from build123d import *

# Parameters (mm, degrees)
SKETCH1_W           = 9.75
SKETCH1_H           = 9.75
SKETCH1_W_2         = 7.75
SKETCH1_H_2         = 7.75
BOSS_EXTRUDE1_DEPTH = 10
BOSS_EXTRUDE2_DEPTH = 4
FILLET1_R           = 1


with BuildPart() as part:
    # Sketch1 → Boss-Extrude1 (new body)
    with BuildSketch(Plane.XY):
        Rectangle(SKETCH1_W, SKETCH1_H)
        Rectangle(SKETCH1_W_2, SKETCH1_H_2, mode=Mode.SUBTRACT)
    extrude(amount=BOSS_EXTRUDE1_DEPTH)

    # Sketch2 → Boss-Extrude2 (add)
    with BuildSketch(Plane.XY.offset(10)):
        with BuildLine():
            Line((-5.253161089, 7.228716278), (5.253161089, 7.228716278))
            ThreePointArc((5.253161089, 7.228716278), (6.667374652, 6.64292984), (7.253161089, 5.228716278))
            Line((7.253161089, 5.228716278), (7.253161089, -5.228716278))
            ThreePointArc((7.253161089, -5.228716278), (6.667374652, -6.64292984), (5.253161089, -7.228716278))
            Line((5.253161089, -7.228716278), (-5.253161089, -7.228716278))
            ThreePointArc((-5.253161089, -7.228716278), (-6.667374652, -6.64292984), (-7.253161089, -5.228716278))
            Line((-7.253161089, -5.228716278), (-7.253161089, 5.228716278))
            ThreePointArc((-7.253161089, 5.228716278), (-6.667374652, 6.64292984), (-5.253161089, 7.228716278))
        make_face()
    extrude(amount=BOSS_EXTRUDE2_DEPTH)

    # Fillet1
    fillet1_edges = [part.edges().sort_by_distance(p)[0] for p in [
        (6.667374652, 6.64292984, 14),
        (0, 7.228716278, 14),
        (-6.667374652, 6.64292984, 14),
        (-7.253161089, 0, 14),
        (-6.667374652, -6.64292984, 14),
        (0, -7.228716278, 14),
        (6.667374652, -6.64292984, 14),
        (7.253161089, 0, 14),
    ]]
    fillet(fillet1_edges, radius=FILLET1_R)


solid = part.part
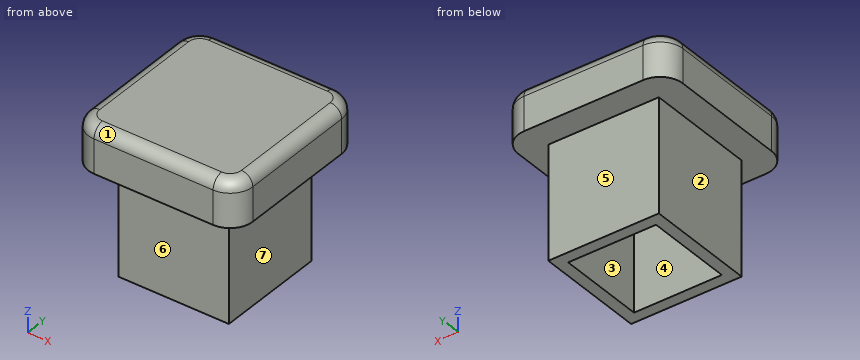
Input: part model. Units: mm. Frame: model coordinates. Face numbers are marked on the shaded views. A direction names the side the tool comes from. Give positions to 0.01 mm unless a question says otherwise; leave off trailing zeros. Loops run counter-clockwise (first coordinate to the right, second up) from the corner with the lowest first, then second, coordinate; pieces in that order, holes last. Notation, with made-up numbers: (24, -5) - (59, -5) arc R35 cw to (59, 31) - close; hole circle Ø5 at (75.5, 27). An arc over 180 degrees is marked (long way). Use CSV: the item, a comma, the result in double quotes. Start each with the question number.
Item 1: Section A-A on z = 5.5. Return loops of the section in (x, y) (3 decimals).
Item 2: Mould query, pull axis X, two halves, no side actions, for the marked faces 1, 2 and 3. Classes: pulls with the +X half, pulls with the -X half, needs draft (parallel to the pull), parting line crosses it, or undercut.
Item 3: Reachability of the marked faces 4, 5, 6 and 7 from +Z, -Z, +X, -X, +Y, -Y: full face, straight path, thin tool, end or side. Return the list, or none.
Item 4: Contact query for flat-ended pins moving along their axis: P1, Ø6, axis at x = 0, z = 2.5, coming from the +Y side (3 decimals); P2, Ø3, axis at y = 0, z = 5.5, coming from the +X side (3 decimals); P3, Ø8, axis at x = 1.5, z = 3, coming from the -Y side (3 decimals). Output: stop coordinate, or through.
Item 5: Section B-B on y = -4.5. Return loops of the section in (x, z) (3 decimals).
Item 6: Section C-C on x = 2.5. Return loops of the section in (y, z) (3 decimals), then the cut area to 3 significant figures.
Item 7: Section D-D on z = 10.25. Return loops of the section in (x, y).
Item 8: Line query: line 1 (X direction, y = -1.5, z = 4) (3 decimals); line 2 (Z direction, x = -0.25, y = 0.25). Output: solid intervals per line, ascending.
Ans:
1,outline,"(-4.875, -4.875) - (4.875, -4.875) - (4.875, 4.875) - (-4.875, 4.875) - close; hole (-3.875, -3.875) - (3.875, -3.875) - (3.875, 3.875) - (-3.875, 3.875) - close"
2,face 1,"needs draft"
2,face 2,"pulls with the -X half"
2,face 3,"undercut"
3,face 4,"-Z"
3,face 5,"-Z, +X, -X, +Y"
3,face 6,"-Z, +X, -X, -Y"
3,face 7,"-Z, +X, +Y, -Y"
4,P1,"stops at y = 4.875"
4,P2,"stops at x = 4.875"
4,P3,"stops at y = -4.875"
5,outline,"(-7.253, 10) - (-4.875, 10) - (-4.875, 0) - (4.875, 0) - (4.875, 10) - (7.253, 10) - (7.253, 13) arc R1 ccw to (6.253, 14) - (-6.253, 14) arc R1 ccw to (-7.253, 13) - close"
6,outline,"(-7.229, 10) - (-4.875, 10) - (-4.875, 0) - (-3.875, 0) - (-3.875, 10) - (3.875, 10) - (3.875, 0) - (4.875, 0) - (4.875, 10) - (7.229, 10) - (7.229, 13) arc R1 ccw to (6.229, 14) - (-6.229, 14) arc R1 ccw to (-7.229, 13) - close"
6,area,"77.4 mm2"
7,outline,"(-7.25, -5.23) arc R2 ccw to (-5.25, -7.23) - (5.25, -7.23) arc R2 ccw to (7.25, -5.23) - (7.25, 5.23) arc R2 ccw to (5.25, 7.23) - (-5.25, 7.23) arc R2 ccw to (-7.25, 5.23) - close"
8,line 1,"x = -4.875 to -3.875, 3.875 to 4.875"
8,line 2,"z = 10 to 14"
